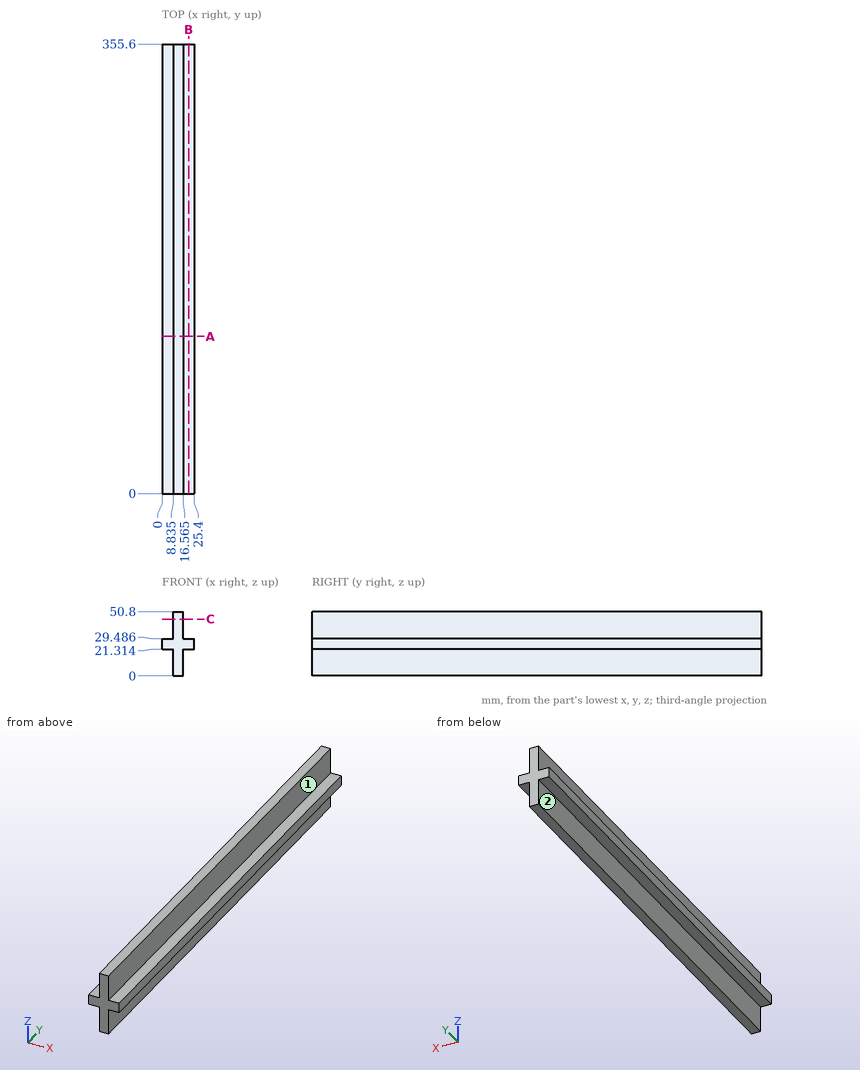
Here's the drawing with two shaded views (mm, measured from the low corner). I have some questions. A direction names the side the tool comes from. Coordinates: 2 decimals unless noted, no trailing zeros. Loops run counter-clockwise (first coordinate to the right, second up) from the corner with the lowest first, then second, coordinate; pieces in that order, holes last. Notation, with made-up numbers: M 60.25,55 L 99.25,55 A20 ccw 99.25,92 Z; hole C 82,50.5 d2. An arc over 180 degrees is marked long. Return JSON: item names as keys, results as strings. Group by question number.
Item 1: Imagine slicing it at C-C (z = 45). Please give me the cut outline in (x, y) (1 decimal), and give its area (3 significant figures).
Item 2: Imagine slicing it at A-A (y = 124.5). Please give me the cut outline in (x, z) (1 decimal), and give its area (3 significant figures).
Item 3: On a 3-axis mill with a long thin cutter (end or side, diameter ignored), from which of +Z, -Z, +X, -X, +Y, -Y can I reach the whole of each face in a straight line? I mean the marked faces 1 and 2. Say none if no direction works.
Item 4: Imagine slicing it at B-B (x = 21). Please give me the cut outline in (y, z).
Item 5: If I drill on L1, parallel to X at y = 314.5, z = 33.5 (1 decimal); L2, parallel to Z at x = 2.5, y = 51, over which ranges is the centre line in solid material (lowest first)? Write a range as from..to.
Item 6: I'm going to push flat-ended pins straight in: pin 1 Ø3 at (x, y) = (4, 232.5) entering from +Z; pin 2 Ø23.5 at (y, z) = (258.5, 9.5) entering from +X (3 decimals); pin 3 Ø4 at (x, y) = (22, 194) entering from -Z. Where does each tip first touch, or does it pass through?
Verdict:
{
 "1": {"outline": "M 8.8,0 L 16.6,0 L 16.6,355.6 L 8.8,355.6 Z", "area": "2,750 mm^2"},
 "2": {"outline": "M 0,21.3 L 8.8,21.3 L 8.8,0 L 16.6,0 L 16.6,21.3 L 25.4,21.3 L 25.4,29.5 L 16.6,29.5 L 16.6,50.8 L 8.8,50.8 L 8.8,29.5 L 0,29.5 Z", "area": "537 mm^2"},
 "3": {"face 1": "+Z, +X, +Y, -Y", "face 2": "-Z, -X, +Y, -Y"},
 "4": {"outline": "M 0,21.31 L 355.6,21.31 L 355.6,29.49 L 0,29.49 Z"},
 "5": {"L1": "x = 8.8..16.6", "L2": "z = 21.31..29.49"},
 "6": {"pin 1": "stops at z = 29.49", "pin 2": "stops at x = 16.565", "pin 3": "stops at z = 21.31"}
}
